Source: CAD feature listing. Evaluate the final solid. Frame: model axes, mm. A direction names the side the tool comes from. Round coordinates to 2 decimals unless told otherwise and drop trailing zeros. Loops run counter-clockwise (first coordinate to the right, second up) from the corner with the lowest first, then second, coordinate; pieces in that order, holes last. Notation, with made-up numbers: (-0.5, 45.5) -> (33.5, 45.5) arc R23 cw to (33.5, 72.5) -> close; hole circle Ø6 at (39.25, 17.5). An arc over 180 degrees is marked (long way). Put each result on its own line as item: value. Start each with the question number.
1. Material intervals for L1, parallel to X at y = 7.95, z = 0; L2, parallel to X at y = 17.75, z = 0; L3, parallel to Y at x = -30.5, z = -14.5, sorted ascending.
2. Cut plane B-B (x = 40). Return the cut outline in (y, z), then the cut area to 3 significant figures.
3. Contact query for flat-ended pins moving along their axis: pin 1 (17 mm diameter, centred on x = 0, z = -40, fed in from +Y); pin 2 (10 mm diameter, centred on x = -8, y = 15.5, fed in from -Z); pin 3 (11.5 mm diameter, centred on x = 40, z = 0, fed in from -Y); pin 4 (13.5 mm diameter, centred on x = -40, z = 0, fed in from +Y). Output: stop coordinate, or through.
4. Cut plane A-A (z = -40). Return the cut outline in (x, y).
5. Draft query along Z for faces 4 (the cylindrical face through (-0.66, 11.042, 14.985)), 5 (the flat face through (7, 1.283, -14)), 6 (the cylindrical face through (-15.02, 13.31, -47.69)). Return one class per face: pulls with the +Z half, pulls with the -Z half, needs draft (parallel to the pull), parting line crosses it, or undercut.
6. Cut plane D-D (z = 0). Return the cut outline in (x, y).
7. Cut plane C-C (y = 9). Return the cut outline in (x, z).
8. Set-up query: faces 1 (the cylindrical face through (-9.76, 3.75, -31)), 2 (the flat face through (40, 11.933, 5)), 3 (the flat face through (-12, 20.533, 10)). Return all of +Z, -Z, +X, -X, +Y, -Y with unobstructed straight access to the full face (end or side cutting, diameter ignored); none if empty.
```python
from build123d import *

# Parameters (mm, degrees)
POG_BIENIE_WALCOWE_POD_M8_WKR_T_Z_BEM_W_D           = 9
POG_BIENIE_WALCOWE_POD_M8_WKR_T_Z_BEM_W_DEPTH       = 42
POG_BIENIE_WALCOWE_POD_M8_WKR_T_Z_BEM_W_CBORE_D     = 15
POG_BIENIE_WALCOWE_POD_M8_WKR_T_Z_BEM_W_CBORE_DEPTH = 8.6
POG_BIENIE_WALCOWE_POD_M8_WKR_T_Z_BEM_W_TIP         = 2.703872786


with BuildPart() as part:
    # Szkic1 → Obrót1 (revolve)
    with BuildSketch(Plane.XY, mode=Mode.PRIVATE) as obr_t1_sk:
        Polygon((-15, 20.532632774), (-50, 20.532632774), (-50, 6.282632774), (-32.5, 6.282632774), (-32.5, 1.282632774), (-15, 1.282632774), align=None)
    revolve(obr_t1_sk.sketch.rotate(Axis((0, 0, 0), (0, 1, 0)), 270), axis=Axis((0, 0, 0), (0, 1, 0)))

    # Pogłębienie walcowe pod M8 Wkręt z łbem walcowym z gniazdem sześciokątnym1
    with Locations(Plane(origin=(-40, 20.532632774, 0), x_dir=(0, 0, 1), z_dir=(0, 1, 0))):
        with Locations((0, 0), (-40, 40), (0, 80), (40, 40)):
            CounterBoreHole(POG_BIENIE_WALCOWE_POD_M8_WKR_T_Z_BEM_W_D / 2, POG_BIENIE_WALCOWE_POD_M8_WKR_T_Z_BEM_W_CBORE_D / 2, POG_BIENIE_WALCOWE_POD_M8_WKR_T_Z_BEM_W_CBORE_DEPTH, depth=POG_BIENIE_WALCOWE_POD_M8_WKR_T_Z_BEM_W_DEPTH)
            with Locations((0, 0, -(POG_BIENIE_WALCOWE_POD_M8_WKR_T_Z_BEM_W_DEPTH + POG_BIENIE_WALCOWE_POD_M8_WKR_T_Z_BEM_W_TIP / 2))):  # 118° drill point
                Cone(0, POG_BIENIE_WALCOWE_POD_M8_WKR_T_Z_BEM_W_D / 2, POG_BIENIE_WALCOWE_POD_M8_WKR_T_Z_BEM_W_TIP, mode=Mode.SUBTRACT)


solid = part.part
```
Solution:
1. L1: x = -50 to -44.5, -35.5 to -15, 15 to 35.5, 44.5 to 50
1. L2: x = -50 to -47.5, -32.5 to -15, 15 to 32.5, 47.5 to 50
1. L3: y = 6.28 to 20.53
2. outline: (6.28, -30) -> (20.53, -30) -> (20.53, -7.5) -> (11.93, -7.5) -> (11.93, -4.5) -> (6.28, -4.5) -> close; (6.28, 4.5) -> (11.93, 4.5) -> (11.93, 7.5) -> (20.53, 7.5) -> (20.53, 30) -> (6.28, 30) -> close
2. area: 675 mm^2
3. pin 1: stops at y = 20.53
3. pin 2: stops at z = -49.91
3. pin 3: stops at y = 6.28
3. pin 4: stops at y = 11.93
4. outline: (-30, 6.28) -> (-4.5, 6.28) -> (-4.5, 11.93) -> (-7.5, 11.93) -> (-7.5, 20.53) -> (-30, 20.53) -> close; (4.5, 6.28) -> (30, 6.28) -> (30, 20.53) -> (7.5, 20.53) -> (7.5, 11.93) -> (4.5, 11.93) -> close
5. face 4: undercut
5. face 5: needs draft
5. face 6: parting line crosses it
6. outline: (-50, 6.28) -> (-44.5, 6.28) -> (-44.5, 11.93) -> (-47.5, 11.93) -> (-47.5, 20.53) -> (-50, 20.53) -> close; (-35.5, 6.28) -> (-32.5, 6.28) -> (-32.5, 1.28) -> (-15, 1.28) -> (-15, 20.53) -> (-32.5, 20.53) -> (-32.5, 11.93) -> (-35.5, 11.93) -> close; (15, 1.28) -> (32.5, 1.28) -> (32.5, 6.28) -> (35.5, 6.28) -> (35.5, 11.93) -> (32.5, 11.93) -> (32.5, 20.53) -> (15, 20.53) -> close; (44.5, 6.28) -> (50, 6.28) -> (50, 20.53) -> (47.5, 20.53) -> (47.5, 11.93) -> (44.5, 11.93) -> close
7. outline: circle Ø100 at (0, 0); hole circle Ø9 at (-40, 0); hole circle Ø30 at (0, 0); hole circle Ø9 at (0, -40); hole circle Ø9 at (0, 40); hole circle Ø9 at (40, 0)
8. face 1: -Y
8. face 2: +Y
8. face 3: +Z, -Z, +X, -X, +Y
